Autodesk Inventor part; units mm, degrees
ref_plane "YZ Plane" through (0, 0, 0) normal (1, 0, 0) x (0, 1, 0)
ref_plane "XZ Plane" through (0, 0, 0) normal (0, 1, 0) x (-1, 0, 0)
ref_plane "XY Plane" through (0, 0, 0) normal (0, 0, 1) x (1, 0, 0)
sketch "Эскиз1" plane through (0, 0, 0) normal (0, 0, 1) x (1, 0, 0)
  line L0 (8.4266, -12.65) -> (-2.5734, -12.65)
  line L1 (-2.5734, -12.65) -> (-2.5734, -47.65)
  line L2 (-2.5734, -47.65) -> (8.4266, -47.65)
  line L3 (8.4266, -47.65) -> (8.4266, -82.9136)
  spline S0 degree 4 poles (2.3773, -93.423) (5.3243, -91.0921) (7.8605, -87.681) (8.4266, -85.6037) (8.4266, -82.9136) knots 0.089011 0.089011 0.089011 0.089011 0.089011 1 1 1 1 1
  spline S1 degree 4 poles (1.3465, -94.1725) (1.6324, -93.9967) (1.8997, -93.813) (2.1479, -93.6217) (2.3773, -93.423) knots 0 0 0 0 0 1 1 1 1 1
  spline S2 degree 4 poles (1.2081, -94.2627) (1.2427, -94.2405) (1.2773, -94.218) (1.3119, -94.1954) (1.3465, -94.1725) knots 0 0 0 0 0 1 1 1 1 1
  spline S3 degree 2 poles (-15.5734, -96.9447) (-3.5967, -97.3511) (1.2081, -94.2627) knots 0 0 0 0.59566 0.59566 0.59566
  line L4 (-125.5734, -96.9447) -> (-15.5734, -96.9447)
  spline S4 degree 2 poles (-125.5734, -96.9447) (-137.55, -97.3511) (-142.3548, -94.2627) knots 0 0 0 0.59566 0.59566 0.59566
  spline S5 degree 4 poles (-142.3548, -94.2627) (-145.6699, -92.132) (-148.8913, -88.0811) (-149.5734, -85.8665) (-149.5734, -82.9136) knots 0 0 0 0 0 1 1 1 1 1
  line L5 (-149.5734, -82.9136) -> (-149.5734, -35.15)
  spline S6 degree 2 poles (-125.5734, 36.6447) (-137.55, 37.0511) (-142.3548, 33.9627) knots 0 0 0 0.59566 0.59566 0.59566
  line L6 (-15.5734, 36.6447) -> (-125.5734, 36.6447)
  spline S7 degree 2 poles (-15.5734, 36.6447) (-3.5967, 37.0511) (1.2081, 33.9627) knots 0 0 0 0.59566 0.59566 0.59566
  spline S8 degree 4 poles (1.2081, 33.9627) (4.5231, 31.832) (7.7445, 27.7811) (8.4266, 25.5665) (8.4266, 22.6136) knots 0 0 0 0 0 1 1 1 1 1
  line L7 (8.4266, 22.6136) -> (8.4266, -12.65)
  line L8 (-10.5734, -92.9447) -> (-10.5734, 32.6447)
  line L9 (-10.5734, 32.6447) -> (-130.5734, 32.6447)
  line L10 (-130.5734, 32.6447) -> (-130.5734, -92.9447)
  line L11 (-130.5734, -92.9447) -> (-10.5734, -92.9447)
  line L12 (5.7794, 10.35) -> (5.7794, -10.35)
  line L13 (-8.4266, 10.35) -> (5.7794, 10.35)
  line L14 (-8.4266, -10.35) -> (-8.4266, 10.35)
  line L15 (5.7794, -10.35) -> (-8.4266, -10.35)
  circle A0 centre (-0.824, -6.35) radius 2.1
  line L16 (-10.5734, 32.6447) -> (-10.5734, -92.9447)
  line L17 (-10.5734, -92.9447) -> (-130.5734, -92.9447)
  line L18 (-130.5734, -92.9447) -> (-130.5734, 32.6447)
  line L19 (-130.5734, 32.6447) -> (-10.5734, 32.6447)
  line L20 (8.4266, -47.65) -> (-2.5734, -47.65)
  line L21 (-2.5734, -47.65) -> (-2.5734, -12.65)
  line L22 (-2.5734, -12.65) -> (8.4266, -12.65)
  line L23 (8.4266, 22.6136) -> (8.4266, -12.65)
  spline S9 degree 4 poles (1.2081, 33.9627) (4.5231, 31.832) (7.7445, 27.7811) (8.4266, 25.5665) (8.4266, 22.6136) knots 0 0 0 0 0 1 1 1 1 1
  spline S10 degree 2 poles (-15.5734, 36.6447) (-3.5967, 37.0511) (1.2081, 33.9627) knots 0 0 0 0.59566 0.59566 0.59566
  line L24 (-125.5734, 36.6447) -> (-15.5734, 36.6447)
  spline S11 degree 2 poles (-142.3548, 33.9627) (-137.55, 37.0511) (-125.5734, 36.6447) knots -0.59566 -0.59566 -0.59566 0 0 0
  spline S12 degree 4 poles (-142.3548, 33.9627) (-145.6699, 31.832) (-148.8913, 27.7811) (-149.5734, 25.5665) (-149.5734, 22.6136) knots 0 0 0 0 0 1 1 1 1 1
  line L25 (-149.5734, 22.6136) -> (-149.5734, -25.15)
  spline S13 degree 2 poles (-125.5734, -96.9447) (-137.55, -97.3511) (-142.3548, -94.2627) knots 0 0 0 0.59566 0.59566 0.59566
  line L26 (-15.5734, -96.9447) -> (-125.5734, -96.9447)
  spline S14 degree 2 poles (-15.5734, -96.9447) (-3.5967, -97.3511) (1.2081, -94.2627) knots 0 0 0 0.59566 0.59566 0.59566
  spline S15 degree 4 poles (1.2081, -94.2627) (1.2427, -94.2405) (1.2773, -94.218) (1.3119, -94.1954) (1.3465, -94.1725) knots 0 0 0 0 0 1 1 1 1 1
  spline S16 degree 4 poles (2.3773, -93.423) (2.1479, -93.6217) (1.8997, -93.813) (1.6324, -93.9967) (1.3465, -94.1725) knots 0 0 0 0 0 1 1 1 1 1
  spline S17 degree 4 poles (2.3773, -93.423) (5.3243, -91.0921) (7.8605, -87.681) (8.4266, -85.6037) (8.4266, -82.9136) knots 0.089011 0.089011 0.089011 0.089011 0.089011 1 1 1 1 1
  line L27 (8.4266, -47.65) -> (8.4266, -82.9136)
  circle A1 centre (-0.824, -6.35) radius 3.8
  line L28 (-0.824, -6.35) -> (0.782, -9.794)
  line L29 (0.782, -9.794) -> (8.4266, -6.2292)
  line L30 (-0.824, -6.35) -> (-0.824, -10.35)
  circle A2 centre (-8.0734, 33.9917) radius 2.5
  line L31 (-8.0734, 33.9917) -> (-7.8457, 36.4813)
  spline S18 degree 4 poles (-8.3011, 31.5021) (-5.572, 31.2525) (-0.0854, 27.7372) (3.5121, 26.3853) (3.4266, 14.7728) (3.4266, 10.35) knots 0 0 0 0 0 0.467272 1 1 1 1 1
  line L32 (8.4266, 10.35) -> (3.4266, 10.35)
  line L33 (-7.8457, 36.4813) -> (-8.3011, 31.5021)
  line L34 (-2.0361, 28.9154) -> (1.2081, 33.9627)
  line L35 (-0.824, -10.15) -> (-7.824, -10.15)
  line L36 (-7.824, -10.15) -> (-7.824, 7.7089)
  line L37 (-7.824, 7.7089) -> (3.4266, 7.7089)
  line L38 (3.4266, 7.7089) -> (3.4266, 10.35)
  line L39 (-8.7741, -6.8356) -> (-1.2266, 9.35)
  line L40 (-8.7741, -6.8356) -> (-2.4299, -9.794)
  line L41 (-1.2266, 9.35) -> (4.6043, 6.631)
  circle A3 centre (-0.824, -6.35) radius 7
  circle A4 centre (-0.824, -6.35) radius 15.7052
  line L42 (-1.2266, 9.35) -> (3.4266, 9.4693)
  circle A5 centre (-0.824, -6.35) radius 1.5
  line L43 (-138.5734, -25.15) -> (-149.5734, -25.15)
  line L44 (-149.5734, -25.15) -> (-149.5734, 22.6136)
  line L45 (-149.5734, -35.15) -> (-138.5734, -35.15)
  line L46 (-138.5734, -35.15) -> (-138.5734, -25.15)
  line L47 (-149.5734, -25.15) -> (-138.5734, -25.15)
  line L48 (-138.5734, -25.15) -> (-138.5734, -35.15)
  line L49 (-138.5734, -35.15) -> (-149.5734, -35.15)
  line L50 (-149.5734, -35.15) -> (-149.5734, -82.9136)
  line L51 (-9.8234, -70.25) -> (-9.8234, -63.25)
  line L52 (-9.8234, -63.25) -> (4.1266, -63.25)
  line L53 (4.1266, -63.25) -> (4.1266, -70.25)
  line L54 (4.1266, -70.25) -> (-9.8234, -70.25)
  line L55 (-9.9734, 2.95) -> (-9.9734, 9.95)
  line L56 (-9.9734, 9.95) -> (4.1266, 9.95)
  line L57 (4.1266, 9.95) -> (4.1266, 2.95)
  line L58 (4.1266, 2.95) -> (-9.9734, 2.95)
  line L59 (-9.8234, -63.25) -> (-9.8234, -70.25)
  line L60 (-9.8234, -70.25) -> (4.1266, -70.25)
  line L61 (4.1266, -70.25) -> (4.1266, -63.25)
  line L62 (4.1266, -63.25) -> (-9.8234, -63.25)
  line L63 (-9.9734, 9.95) -> (-9.9734, 2.95)
  line L64 (-9.9734, 2.95) -> (4.1266, 2.95)
  line L65 (4.1266, 2.95) -> (4.1266, 9.95)
  line L66 (4.1266, 9.95) -> (-9.9734, 9.95)
  spline S19 degree 4 poles (-142.3548, -94.2627) (-145.6699, -92.132) (-148.8913, -88.0811) (-149.5734, -85.8665) (-149.5734, -82.9136) knots 0 0 0 0 0 1 1 1 1 1
  spline S20 degree 4 poles (-142.3548, 33.9627) (-145.6699, 31.832) (-148.8913, 27.7811) (-149.5734, 25.5665) (-149.5734, 22.6136) knots 0 0 0 0 0 1 1 1 1 1
  point P0 (0, 0)
  point P1 (1.9242, 24.3867)
  point P2 (3.4266, 9.35)
  point P3 (-6.5685, -10.35)
  point P4 (5.7794, -8.6727)
  point P5 (6.11, -7.3095)
  point P6 (-7.886, 36.4854)
  point P7 (-7.824, -6.35)
  point P8 (-6.7027, -10.15)
  point P9 (-7.8466, 36.4837)
  point P10 (1.2103, 33.9674)
  point P11 (-7.8461, 36.4827)
  point P12 (1.2099, 33.9666)
  point P13 (-7.8465, 36.4834)
  point P14 (-7.8062, 36.4797)
  point P15 (1.2097, 33.9661)
  point P16 (-7.8463, 36.4828)
  point P17 (-7.8061, 36.4794)
  point P18 (1.2094, 33.9656)
  point P19 (-7.8462, 36.4824)
  point P20 (-7.846, 36.4824)
  point P21 (-7.8462, 36.4824)
  point P22 (1.2092, 33.9651)
  point P23 (-7.8457, 36.4813)
  point P24 (1.2089, 33.9645)
  point P25 (-7.8461, 36.4821)
  point P26 (-7.8058, 36.4784)
  point P27 (1.2087, 33.964)
  point P28 (-7.8458, 36.4813)
  point P29 (-7.8057, 36.4781)
  point P30 (1.2085, 33.9635)
  point P31 (-7.8458, 36.4813)
  point P32 (-7.8457, 36.4813)
  dimension "d0" = 7.6
  dimension "d1" = 25
  dimension "d2" = 5
  dimension "d3" = 5
  dimension "d4" = 6
  dimension "d6" = 7
  dimension "d7" = 25
  dimension "d8" = 7
  dimension "d9" = 1
  dimension "d13" = 3
extrude "Выдавливание1" add sketch "Эскиз1" along normal blind 2 contours L29 A3 L12 A4 L7 | A4 L12 L32 L7 | L29 L12 A3 | L32 L13 S18 L34 S8 L7 | A4 L57 L56 L38 L13 L12 | L12 A3 L39 L58 L57 A4 | L29 A1 L40 A3 L12 | A3 L40 A1 L35 | L30 A0 L28 A1 | A1 L28 A0 L30 | L57 L41 L37 L38 A4 | A4 L38 L56 L57 | L30 A5 L28 A0 | A0 L28 A5 L30 | L34 S18 A2 S7 | A3 L36 L39 | L39 L36 L58 | A4 L42 L38 | L38 L37 L41 A4 | L57 L58 L39 L37 L41 | L31 L33 A2 | A2 L33 L31 | L58 L36 L37 L39 | L41 L37 L39 | L39 L37 A4 picked at (5.8525, -5.4253)
sketch "Эскиз2" plane through (0, 0, 2) normal (0, 0, 1) x (1, 0, 0)
  line L0 (8.4266, -6.2292) -> (8.4266, 22.6136)
  line L1 (0.782, -9.794) -> (8.4266, -6.2292)
  arc A0 (-0.824, -10.15) -> (0.782, -9.794) centre (-0.824, -6.35) ccw
  line L2 (-6.7027, -10.15) -> (-0.824, -10.15)
  arc A1 (-7.824, -6.35) -> (-6.7027, -10.15) centre (-0.824, -6.35) ccw
  line L3 (-7.824, 7.7089) -> (-7.824, -6.35)
  arc A2 (-1.2266, 9.35) -> (-7.824, 7.7089) centre (-0.824, -6.35) ccw
  line L4 (3.4266, 9.4693) -> (-1.2266, 9.35)
  line L5 (3.4266, 10.35) -> (3.4266, 9.4693)
  arc A3 (-7.8457, 36.4813) -> (-8.3011, 31.5021) centre (-8.0734, 33.9917) ccw
  circle A4 centre (-0.824, -6.35) radius 1.5
  circle A5 centre (-0.824, -6.35) radius 43.4879
  arc A6 (-7.8458, 36.4818) -> (-8.3011, 31.5021) centre (-8.0734, 33.9917) ccw
  point P0 (0, 0)
  point P1 (-7.8466, 36.4842)
  point P2 (-7.8463, 36.4831)
properties part number "limit_arm"
Input: part model. Units: mm. Frame: model coordinates. A direction names the side the tool comes from. Coordinates: 2 decimals unless noted, no trailing zeros. Write each loop counter-clockwise with the first axis right and the second up, starting at its lowest first coordinate (ties: lowest second). Pieces come first, ordered by that corner, then holes. Notation, with made-up numbers: M -33,7 L 6,7 A21 cw 6,14 Z; hole C 12.5,57.25 d11. An arc over 180 degrees is marked long. Use one line per item in the form item = value.
Q1. Material intervals for probe 1 along Y at (x, z) = (-1.5, 0.95); probe 2 along X at (y, z) = (0, 1.85); probe 3 along X at (y, z) = (12.5, 1.8), sorted ascending. Write a range as from..to.
Answer below:
probe_1 = -10.15..-7.69, -5.01..9.34, 28.54..35.24
probe_2 = -7.82..8.43
probe_3 = 3.42..8.43
Q2. Draft query along Y for faces 1 (the face through (8.427, 8, 1)), 2 (the face through (-10.567, 34.165, 0.986)), 3 (the face through (3.427, 10, 1)). Return one class per face: released by +Y, released by -Y, zero draft, split by the parting line, or undercut.
Answer below:
face_1 = zero draft
face_2 = split by the parting line
face_3 = undercut
Q3. Set-up query: faces 4 (the face through (-7.824, 1, 1)), 5 (the face through (0.01, -10.057, 0.986)), 6 (the face through (-4.66, 8.88, 0.99)). Return all of +Z, -Z, +X, -X, +Y, -Y with unobstructed straight access to the full face (end or side cutting, diameter ignored); none if empty.
Answer below:
face_4 = +Z, -Z, -X, -Y
face_5 = +Z, -Z, +X, -Y
face_6 = +Z, -Z, -X
Q4. Section A-A (x = -9). Return loops of the section in (y, z).
Answer below:
outline = M 31.67,0 L 36.31,0 L 36.31,2 L 31.67,2 Z
